For this review, take the finished solid that the model builds, in its own axes (mm). A direction names the side the tool comes from. Coordinates: 2 decimals unless noted, no trailing zeros. Order: outer loops, then holes, each group sorted by start corner. A loop starts at its lowest first (then second) coordinate and runs counter-clockwise, first axis right, second up. Notation, with made-up numbers: (67.25, 10) - (95.25, 10) arc R28 ccw to (95.25, 32) - close; hole circle Ø5 at (7, -19). An arc over 180 degrees is marked (long way). One line per item, written item: value. Start each with the question number.
(1) Mouldability with a two-part tool opening along X and no side actions: class faces 1 (the flat face through (0, -5, -4)), 2 (the flat face through (-39.96, -4.93, 16.83)), 3 (the flat face through (39.96, -4.93, -16.83)) as released by +X, released by -X, zero draft, split by the parting line, or undercut.
(2) Clearance check with flat-ended pins moving along their axes: pin 1 (3 mm diameter, centred on y = -2, z = -15.5, fed in from +X); pin 2 (2.5 mm diameter, centred on y = -3.5, z = -1.5, fed in from -X); pin 3 (5 mm diameter, centred on y = -5, z = -10, fed in from -X). State where each tip first meets the part, or that it passes through.
(3) Consider section A-A on y = -7.75. Write out the cut boundary in (x, z).
(4) To check wall thickness, follow line 1 along Z through (x, y) = (-18, -2.25); line 2 along X through (y, z) = (-8.75, -1); line 3 along Z through (x, y) = (10, -8.5). State the ranges of each line that lie inside material, in increasing order.
(5) Consider section B-B on x = -12. Write out the cut boundary in (y, z), then the cut area to 3 significant figures.
(6) For faces 4 (the flat face through (16.36, -4.93, -40.155)), 5 (the flat face through (20, -5, 0)), list the 3-axis set-ups (+Z, -Z, +X, -X, +Y, -Y) from which the entire face can be reached by the end or side of a thin tool; tool diameter is ignored.
(7) Consider section D-D on x = 4.5. Write out the cut boundary in (y, z), then the cut area to 3 significant figures.
(8) Consider section C-C on z = -6.5. Write out the cut boundary in (x, y), then the cut area to 3 significant figures.
```python
from build123d import *

# Parameters (mm, degrees)
F1_DEPTH = 10


with BuildPart() as f1:
    # F0 (on Front) → F1 (new body)
    with BuildSketch(Plane.XZ):
        Polygon((-33.185543, 33.185543), (-46.931445, 0), (-33.185543, -33.185543), (0, -46.931445), (33.185543, -33.185543), (46.931445, 0), (33.185543, 33.185543), (0, 46.931445), align=None)
        Polygon((-20, -4), (-20, 0), (-20, 4), (0, 4), (20, 4), (20, 0), (20, -4), (0, -4), align=None, mode=Mode.SUBTRACT)
    extrude(amount=F1_DEPTH)


solid = f1.part
```
Geometry check:
1. face 1: undercut
1. face 2: released by -X
1. face 3: released by +X
2. pin 1: stops at x = 41.13
2. pin 2: stops at x = -46.83
2. pin 3: stops at x = -43.82
3. outline: (-46.93, 0) - (-33.19, -33.19) - (0, -46.93) - (33.19, -33.19) - (46.93, 0) - (33.19, 33.19) - (0, 46.93) - (-33.19, 33.19) - close; hole (-20, -4) - (20, -4) - (20, 4) - (-20, 4) - close
4. line 1: z = -39.48 to -4, 4 to 39.48
4. line 2: x = -46.52 to -20, 20 to 46.52
4. line 3: z = -42.79 to -4, 4 to 42.79
5. outline: (-10, -41.96) - (0, -41.96) - (0, -4) - (-10, -4) - close; (-10, 4) - (0, 4) - (0, 41.96) - (-10, 41.96) - close
5. area: 759 mm^2
6. face 4: -Z, +X, +Y, -Y
6. face 5: +Y, -Y
7. outline: (-10, -45.07) - (0, -45.07) - (0, -4) - (-10, -4) - close; (-10, 4) - (0, 4) - (0, 45.07) - (-10, 45.07) - close
7. area: 821 mm^2
8. outline: (-44.24, -10) - (44.24, -10) - (44.24, 0) - (-44.24, 0) - close
8. area: 885 mm^2
